Read the model definition and answer for the solid it produces. Units are mm, in the model's axes. Face numbers are marked on the shaded views. A direction names the side the tool comes from. Round coordinates to 2 decimals unless told otherwise and drop trailing zeros. Order: outer loops, then holes, each group sorted by start corner. A loop starts at its lowest first (then second) coordinate and runs counter-clockwise, first axis right, second up.
from build123d import *

# Parameters (mm, degrees)
F0_W     = 584.2
F0_H     = 28.575
F0_W_2   = 28.575
F0_H_2   = 584.2
F1_DEPTH = 1035.05


with BuildPart() as f1:
    # F0 (on Top) → F1 (new body)
    with BuildSketch(Plane.XY):
        with Locations((12.7, 747.7125)):
            Rectangle(F0_W, F0_H)
        Polygon((-279.4, 733.425), (-279.4, 762), (-304.8, 762), (-304.8, -152.4), (-279.4, -152.4), align=None)
        with BuildLine():
            Line((-279.4, -152.4), (-304.8, -152.4))
            ThreePointArc((-304.8, -152.4), (-126.2522938113, -583.4522938113), (304.8, -762))
            Line((304.8, -762), (304.8, -736.6))
            ThreePointArc((304.8, -736.6), (-108.2917815692, -565.4917815692), (-279.4, -152.4))
        make_face()
        Polygon((304.8, -736.6), (304.8, -762), (1219.2, -762), (1219.2, -736.6), (1190.625, -736.6), align=None)
        with Locations((1204.9125, -444.5)):
            Rectangle(F0_W_2, F0_H_2)
    extrude(amount=F1_DEPTH)


solid = f1.part
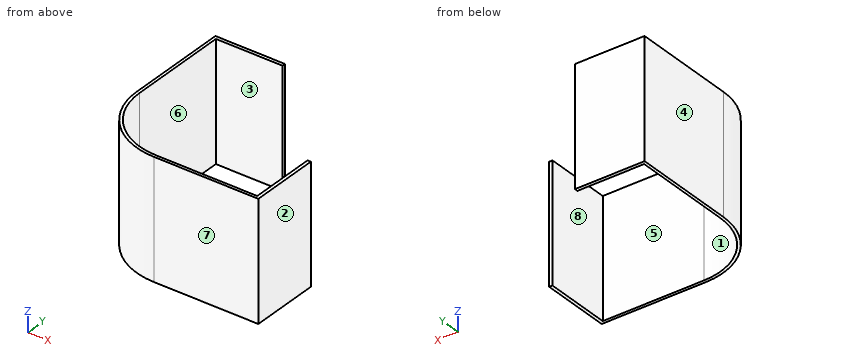
Q1. A cutting plane is placed at B-B, the plane z = 144. Give the vertices of the cut face in (x, y) (3 decimals).
Outcome:
outline: (-304.8, -152.4) arc R609.6 ccw to (304.8, -762) - (1219.2, -762) - (1219.2, -152.4) - (1190.625, -152.4) - (1190.625, -736.6) - (304.8, -736.6) arc R584.2 cw to (-279.4, -152.4) - (-279.4, 733.425) - (304.8, 733.425) - (304.8, 762) - (-304.8, 762) - close
Q2. Straight lines are drawn through the part: probe 1 along X at (y, z) = (596.5, 116); probe 2 along Y at (x, z) = (1028.5, 581); probe 3 along X at (y, z) = (-486.5, 802) (1 decimal). For each, find the intervals that lie inside material, in ascending order.
Outcome:
probe 1: x = -304.8 to -279.4
probe 2: y = -762 to -736.6
probe 3: x = -205.1 to -174.4, 1190.6 to 1219.2
Q3. For the marked faces 1, 2, 3, 4 and 5, determine the directions among +Z, -Z, +X, -X, +Y, -Y from which every point of the face is accessible in a straight line to the end or side of a thin tool.
Outcome:
face 1: +Z, -Z
face 2: +Z, -Z, +X, +Y, -Y
face 3: +Z, -Z, +X
face 4: +Z, -Z, -X, +Y, -Y
face 5: +Z, -Z, +Y
Q4. A cutting plane is placed at C-C, the plane y = -636. Give the vertices of the cut face in (x, z) (3 decimals), plus the area to 3 significant figures.
Outcome:
outline: (-66.338, 0) - (-22.951, 0) - (-22.951, 1035.05) - (-66.338, 1035.05) - close; (1190.625, 0) - (1219.2, 0) - (1219.2, 1035.05) - (1190.625, 1035.05) - close
area: 74,500 mm2
Q5. For a pull along X with two mould halves and no side action, classify the marked faces 6, 7 and 8 as released by +X, released by -X, zero draft, split by the parting line, or undercut.
Outcome:
face 6: released by +X
face 7: zero draft
face 8: undercut
Q6. Flat-ended cylindrical pins translate along their axes: pin 1 (8.5 mm diameter, centred on x = 1202, z = 354, fed in from +Y); pin 2 (1 mm diameter, centred on y = -553, z = 816.5, fed in from -X); pin 3 (8.5 mm diameter, centred on y = 753, z = 693.5, fed in from +X). Find the tip coordinate at first contact, or state that the pin passes through.
Outcome:
pin 1: stops at y = -152.4
pin 2: stops at x = -155.13
pin 3: stops at x = 304.8
Q7. A cutting plane is placed at D-D, the plane y = 192. Give the vertices of the cut face in (x, z), plus the area to 3 significant figures.
Outcome:
outline: (-304.8, 0) - (-279.4, 0) - (-279.4, 1035.05) - (-304.8, 1035.05) - close
area: 26,300 mm2
Q8. A cutting plane is placed at A-A, the plane x = 139.5. Give the vertices of the cut face in (y, z) (3 decimals).
Outcome:
outline: (-739.161, 0) - (-712.726, 0) - (-712.726, 1035.05) - (-739.161, 1035.05) - close; (733.425, 0) - (762, 0) - (762, 1035.05) - (733.425, 1035.05) - close
